```python
from build123d import *

# Parameters (mm, degrees)
SKETCH1_R           = 1.5
BOSS_EXTRUDE1_DEPTH = 3
SKETCH2_R           = 3
BOSS_EXTRUDE2_DEPTH = 1.5
SKETCH3_R           = 2.4
BOSS_EXTRUDE3_DEPTH = 4
SKETCH4_R           = 1.5
BOSS_EXTRUDE4_DEPTH = 10
FILLET1_R           = 20
FILLET2_R           = 2
CUT_EXTRUDE1_DEPTH  = 25.15


with BuildPart() as part:
    # Sketch1 → Boss-Extrude1 (new body)
    with BuildSketch(Plane.XY):
        with BuildLine():
            Line((-12.031480134, -15.968369445), (-10.412459505, -3.978677815))
            ThreePointArc((-10.412459505, -3.978677815), (-6.186542438, -1.207286803), (-8.04761466, 3.491159046))
            Line((-8.04761466, 3.491159046), (-20.07857801, 10.219318997))
            ThreePointArc((-20.07857801, 10.219318997), (-22.325493603, 12.420556624), (-23.15, 15.456057566))
            Line((-23.15, 15.456057566), (-23.15, 32))
            Line((-23.15, 32), (-30.15, 32))
            Line((-30.15, 32), (-30.15, 2.874544331))
            Line((-30.15, 2.874544331), (-18.531088913, -17.25))
            ThreePointArc((-18.531088913, -17.25), (-14.822887986, -18.933878175), (-12.031480134, -15.968369445))
        make_face()
        with Locations((-15.5, -15.5)):
            Circle(SKETCH1_R, mode=Mode.SUBTRACT)
    extrude(amount=BOSS_EXTRUDE1_DEPTH)

    # Sketch2 → Boss-Extrude2 (add)
    with BuildSketch(Plane.XY.offset(3)):
        with Locations((-10, 0)):
            Circle(SKETCH2_R)
    extrude(amount=BOSS_EXTRUDE2_DEPTH)

    # Sketch3 → Boss-Extrude3 (add)
    with BuildSketch(Plane.XY.offset(4.5)):
        with Locations((-10, 0)):
            Circle(SKETCH3_R)
    extrude(amount=BOSS_EXTRUDE3_DEPTH)

    # Sketch4 → Boss-Extrude4 (add)
    with BuildSketch(Plane.XY.offset(3)):
        with BuildLine():
            Line((-12.031480134, -15.968369445), (-10.680184518, -5.96132108))
            ThreePointArc((-10.680184518, -5.96132108), (-15.964537986, -0.651372866), (-11.950849133, 5.673992215))
            Line((-11.950849133, 5.673992215), (-20.07857801, 10.219318997))
            ThreePointArc((-20.07857801, 10.219318997), (-22.325493603, 12.420556624), (-23.15, 15.456057566))
            Line((-23.15, 15.456057566), (-23.15, 32))
            Line((-23.15, 32), (-30.15, 32))
            Line((-30.15, 32), (-30.15, 2.874544331))
            Line((-30.15, 2.874544331), (-18.531088913, -17.25))
            ThreePointArc((-18.531088913, -17.25), (-14.822887986, -18.933878175), (-12.031480134, -15.968369445))
        make_face()
        with Locations((-15.5, -15.5)):
            Circle(SKETCH4_R, mode=Mode.SUBTRACT)
    extrude(amount=BOSS_EXTRUDE4_DEPTH)

    # Fillet1
    fillet1_edges = [part.edges().sort_by_distance(p)[0] for p in [
        (-30.15, 2.874544331, 6.5),
    ]]
    fillet(fillet1_edges, radius=FILLET1_R)

    # Fillet2
    fillet2_edges = [part.edges().sort_by_distance(p)[0] for p in [
        (-30.15, 32, 6.5),
        (-23.15, 32, 6.5),
    ]]
    fillet(fillet2_edges, radius=FILLET2_R)

    # Sketch5 → Cut-Extrude1 (cut, through all)
    with BuildSketch(Plane.ZY.offset(30.15)):
        with BuildLine():
            Line((8.55, 26.75), (8.55, 22.75))
            ThreePointArc((8.55, 22.75), (6.5, 20.7), (4.45, 22.75))
            Line((4.45, 22.75), (4.45, 26.75))
            ThreePointArc((4.45, 26.75), (6.5, 28.8), (8.55, 26.75))
        make_face()
    extrude(amount=-CUT_EXTRUDE1_DEPTH, mode=Mode.SUBTRACT)


solid = part.part
```
Geometry check sheet. Reference: the model listing, model coordinates, mm. A direction names the side the tool comes from. Give positions to 0.01 mm unless a question says otherwise; leave off trailing zeros. Order: outer loops, then holes, each group sorted by start corner. A loop starts at its lowest first (then second) coordinate and runs counter-clockwise, first axis right, second up.
1. Section check D-D, the plane x = -22. Enter the section's corners in (y, z).
2. Thickness scan on L1, parallel to Y at x = -15.5, z = 8.75; L2, parallel to Y at x = -12.5, z = 3.5; L3, parallel to Z at x = -13.5, y = -3.5. Record the ranges inside material, lowest first.
3. Section check B-B, the plane x = -15.5. Enter the section's corners in (y, z).
4. Section check C-C, the plane y = -5. Enter the section's corners in (x, z), and give its area (3 significant figures).
5. Section check A-A, the plane z = 5.25. Enter the section's corners in (x, y), and give its area (3 significant figures).
6. Gauge pin test, flat ends, axial feed: pin 1 Ø2.5 at (x, y) = (-10.5, 0.5) entering from +Z; pin 2 Ø1.5 at (y, z) = (-2, 3) entering from +X; pin 3 Ø4 at (x, z) = (-23.5, 4.5) entering from -Y. Record the tip position at first contact, or that the pin passes through.
7. Release check for a two-part mould opening along X. For faces 4 (the face through (-29.487, 3.128, 6.409)), 5 (the face through (-22.3, 12.38, 6.41)), 6 (the face through (-12.4, -1.8, 3.7)) record: pulls with the +X half, pulls with the -X half, needs draft (parallel to the pull), parting line crosses it, or undercut.
8. Access from +Z, -Z, +X, -X, +Y, -Y to the whole of each face (thin tool, end or side, straight path). Record for faces 1 (the face through (-23.75, 31.43, 6.41)), 2 (the face through (-15.95, -0.76, 7.93)), 3 (the face through (-27, 25, 8.55)).
Values follow:
1. outline: (-11.24, 0) - (11.92, 0) - (11.92, 13) - (-11.24, 13) - close
2. L1: y = -19 to -17, -14 to -2.4, 2.4 to 7.66
2. L2: y = -17.3 to -5.45, -1.66 to 1.66, 5.45 to 5.98
2. L3: z = 0 to 3
3. outline: (-19, 0) - (-17, 0) - (-17, 13) - (-19, 13) - close; (-14, 0) - (7.66, 0) - (7.66, 13) - (2.4, 13) - (2.4, 3) - (-2.4, 3) - (-2.4, 13) - (-14, 13) - close
4. outline: (-25.6, 0) - (-10.55, 0) - (-10.55, 3) - (-13.32, 3) - (-13.32, 13) - (-25.6, 13) - close
4. area: 168 mm2
5. outline: (-30.15, 8.23) arc R20 ccw to (-27.47, -1.77) - (-18.53, -17.25) arc R3.5 ccw to (-12.03, -15.97) - (-10.68, -5.96) arc R6 cw to (-11.95, 5.67) - (-20.08, 10.22) arc R6 cw to (-23.15, 15.46) - (-23.15, 21.13) - (-30.15, 21.13) - close; (-30.15, 28.37) - (-23.15, 28.37) - (-23.15, 30) arc R2 ccw to (-25.15, 32) - (-28.15, 32) arc R2 ccw to (-30.15, 30) - close; circle Ø4.8 at (-10, 0); hole circle Ø3 at (-15.5, -15.5)
5. area: 458 mm2
6. pin 1: stops at z = 8.5
6. pin 2: stops at x = -6.2
6. pin 3: stops at y = -12.11
7. face 4: pulls with the -X half
7. face 5: pulls with the +X half
7. face 6: undercut
8. face 1: +Z, -Z, +X, +Y
8. face 2: +Z
8. face 3: +X, -X
